Autodesk Inventor part; units mm, degrees
ref_plane "YZ Plane" through (0, 0, 0) normal (1, 0, 0) x (0, 1, 0)
ref_plane "XZ Plane" through (0, 0, 0) normal (0, 1, 0) x (-1, 0, 0)
ref_plane "XY Plane" through (0, 0, 0) normal (0, 0, 1) x (1, 0, 0)
sketch "Sketch1" plane through (0, 0, 0) normal (0, 1, 0) x (-1, 0, 0)
  line L0 (0, 0) -> (50, 0)
  line L1 (50, 0) -> (50, -50)
  line L2 (50, -50) -> (0, -50)
  line L3 (0, -50) -> (0, 0)
  circle A0 centre (37.6883, -4.8163) radius 2.5
  circle A1 centre (37.6883, -43.3405) radius 2.5
  circle A2 centre (6.6955, -43.3405) radius 2.5
  circle A3 centre (6.6955, -4.8163) radius 2.5
  dimension "d0" = 50
  dimension "d1" = 50
  dimension "d6" = 5
  dimension "d9" = 5
  dimension "d10" = 5
  dimension "d11" = 5
  dimension "d20" = 25.9928
  dimension "d21" = 38.5242
extrude "Extrusion1" add sketch "Sketch1" along normal blind 80 contours L0 L1 L2 L3 | A0 | A1 | A2 | A3
sketch "Sketch2" plane through (0, 80, 0) normal (0, 1, 0) x (1, 0, 0)
  line L0 (-47.6071, 46.9807) -> (-2.1924, 46.9807)
  line L1 (-2.1924, 46.9807) -> (-2.1924, 2.5056)
  line L2 (-2.1924, 2.5056) -> (-47.6071, 2.5056)
  line L3 (-47.6071, 2.5056) -> (-47.6071, 46.9807)
  point P0 (0, 0)
extrude "Extrusion2" cut sketch "Sketch2" against normal blind 48
extrude "Extrusion3" add sketch "Sketch1" against normal blind 30 contours A0 | A1 | A2 | A3
sketch "Sketch6" plane through (0, 0, 0) normal (1, 0, 0) x (0, 0, -1)
  circle A0 centre (27.1417, 30.3837) radius 2.5
  point P0 (0, 0)
  dimension "d22" = 5
extrude "Extrusion6" add sketch "Sketch6" along normal blind 180
properties part number "Water tank"
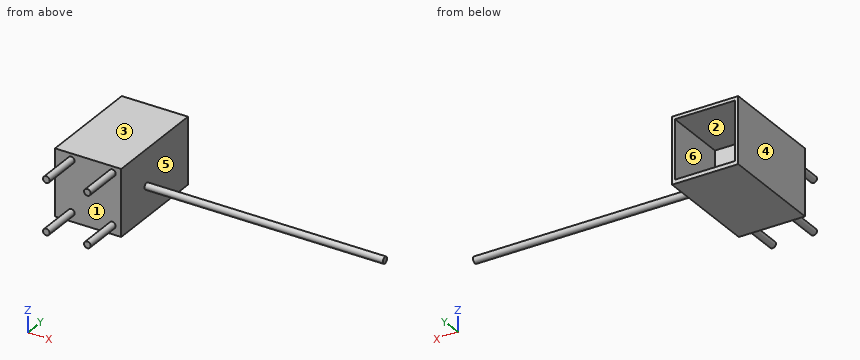
Verification items for the finished model (mm, model axes). Face numbers are marked on the shaded views. A direction names the side the tool comes from. Round coordinates to 2 decimals unless told otherwise and drop trailing zeros. Loops run counter-clockwise (first coordinate to the right, second up) from the corner with the lowest first, then second, coordinate; pieces in that order, holes last. Notation, with made-up numbers: (-2, -7) - (39, -7) arc R29 cw to (39, 27) - close; hole circle Ø3 at (56, 43.25). An arc over 180 degrees is marked (long way). Answer in a Markdown table with one row per item. Add a question column.
Q1. Material ranges on line 1 (X direction, y = 51.5, z = -45.5); line 2 (Z direction, x = -19.5, y = 69.5); line 3 (X direction, y = -6, z = -43.5), recorded low to high.
Q2. Tool access check on the marked faces 1, 2 and 3. Record the directions out of +Z, -Z, +X, -X, +Y, -Y that give a thin tool (end or side, any length) a straight path to the whole face; none if there is none.
Q3. Release check for a two-part mould opening along X. For the marked faces 4, 5 and 6 record: pulls with the +X half, pulls with the -X half, needs draft (parallel to the pull), parting line crosses it, or undercut.
Q4. Section check D-D on y = 4. Enter the section's corners in (x, z).
Q5. Gauge pin test, flat ends, axial feed: pin 1 (1 mm diameter, centred on y = 17.5, z = -5, fed in from +X); pin 2 (13.5 mm diameter, centred on x = -17, z = -20, fed in from +Y); pin 3 (15 mm diameter, centred on x = -30.5, z = -29.5, fed in from -Y). Record the tip position at first contact, or that the pin passes through.
Q6. Section check A-A on z = -20.5. Enter the section's corners in (x, y).
Q7. Section check C-C on x = -27. Enter the section's corners in (y, z).
Q8. Section check B-B on y = 67. Enter the section's corners in (x, z), plus the area to 3 significant figures.
Found:
| question | item | result |
|---|---|---|
| 1 | line 1 | x = -50 to -47.61, -2.19 to 0 |
| 1 | line 2 | z = -50 to -46.98, -2.51 to 0 |
| 1 | line 3 | x = -40.18 to -35.19, -9.19 to -4.2 |
| 2 | face 1 | -Y |
| 2 | face 2 | +Y |
| 2 | face 3 | +Z, +X, -X, +Y, -Y |
| 3 | face 4 | pulls with the -X half |
| 3 | face 5 | pulls with the +X half |
| 3 | face 6 | undercut |
| 4 | outline | (-50, -50) - (0, -50) - (0, 0) - (-50, 0) - close |
| 5 | pin 1 | stops at x = 0 |
| 5 | pin 2 | stops at y = 32 |
| 5 | pin 3 | stops at y = 0 |
| 6 | outline | (-50, 0) - (0, 0) - (0, 80) - (-2.19, 80) - (-2.19, 32) - (-47.61, 32) - (-47.61, 80) - (-50, 80) - close |
| 7 | outline | (0, -50) - (80, -50) - (80, -46.98) - (32, -46.98) - (32, -2.51) - (80, -2.51) - (80, 0) - (0, 0) - close |
| 8 | outline | (-50, -50) - (0, -50) - (0, 0) - (-50, 0) - close; hole (-47.61, -46.98) - (-2.19, -46.98) - (-2.19, -2.51) - (-47.61, -2.51) - close |
| 8 | area | 480 mm² |
